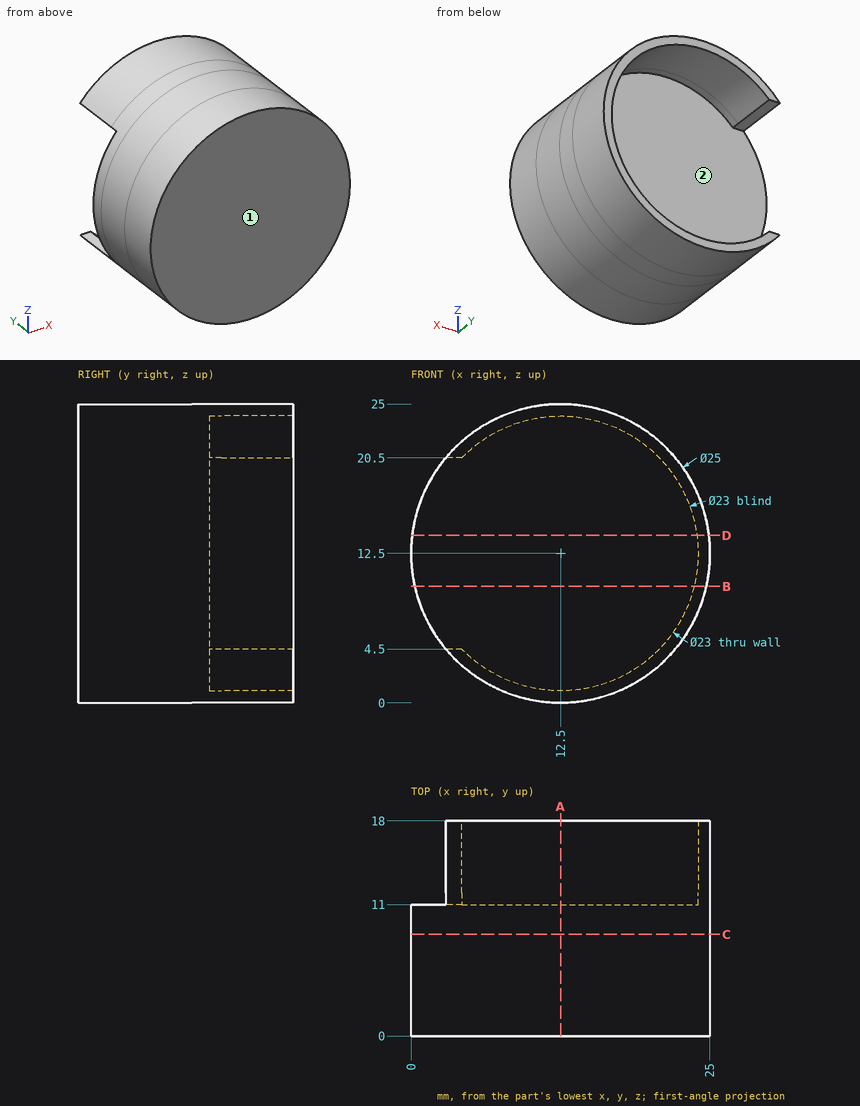
Drawing for the job (mm, zero at the part's lowest x, y, z). Round coordinates to 2 decimals unless told otherwise and drop trailing zeros. Loops run counter-clockwise (first coordinate to the right, second up) from the corner with the lowest first, then second, coordinate; pieces in that order, holes last. Notation, with made-up numbers: (89, -37) -> (125, -37) arc R10 cw to (125, -23) -> close; hole circle Ø11 at (3.25, -26.75). An arc over 180 degrees is marked (long way). Answer as CSV lines item,"result". Start each with the question number.
1) Slice it at C-C (y = 8.5). List the corners of the cut face in (x, z), plus the area to 3 significant figures.
2) Pin check, flat tips, straight feed: P1, Ø2, axis at x = 20, y = 15, coming from the +Z side; P2, Ø1.5, axis at x = 3.5, y = 14.5, coming from the -Z side; P3, Ø1, axis at x = 9.5, y = 13, coming from the +Z side. Stop position of each tip, or through.
3) Probe line 1 along Z through (x, y) = (12.5, 14.85); line 2 along Y through (x, z) = (6.5, 16.25); line 3 along Z through (x, y) = (21.5, 14.5) (1 decimal). List the from-to ranges inside material, lowest first.
4) Slice it at A-A (x = 12.5). List the corners of the cut face in (y, z), plus the area to 3 significant figures.
5) Mould opens along Z. For the marked faces 1 and 2 say: +Z half, -Z half, draft (parallel to the pull), parting line (faces both ways), or undercut.
6) Slice it at B-B (z = 9.75). List the corners of the cut face in (x, y), plus the area to 3 significant figures.
7) Slice it at D-D (z = 14). List the corners of the cut face in (x, y).
Filled in:
1,outline,"circle Ø25 at (12.5, 12.5)"
1,area,"491 mm2"
2,P1,"stops at z = 23.18"
2,P2,"stops at z = 3.11"
2,P3,"stops at z = 24.75"
3,line 1,"z = 0 to 1, 24 to 25"
3,line 2,"y = 0 to 11"
3,line 3,"z = 3.8 to 5.3, 19.7 to 21.2"
4,outline,"(0, 0) -> (18, 0) -> (18, 1) -> (11, 1) -> (11, 24) -> (18, 24) -> (18, 25) -> (0, 25) -> close"
4,area,"289 mm2"
5,face 1,"draft"
5,face 2,"undercut"
6,outline,"(0.31, 0) -> (24.69, 0) -> (24.69, 18) -> (23.67, 18) -> (23.67, 11) -> (0.31, 11) -> close"
6,area,"275 mm2"
7,outline,"(0.09, 0) -> (24.91, 0) -> (24.91, 18) -> (23.9, 18) -> (23.9, 11) -> (0.09, 11) -> close"
